Study the drawing (mm; zero at the part's minimum x, y, z) and answer. Coordinates: 2 decimals unless noted, no trailing zeros. Loops run counter-clockwise (first coordinate to the right, second up) from the corner with the lowest first, then second, coordinate; pieces in that order, holes last. Notation, with made-up numbers: (24, -31) -> (28, -31) arc R8 ccw to (28, -19) -> close; hole circle Ø2 at (3, 10.25). An arc over 180 degrees is marked (long way). Answer in a Markdown table with one row per item.
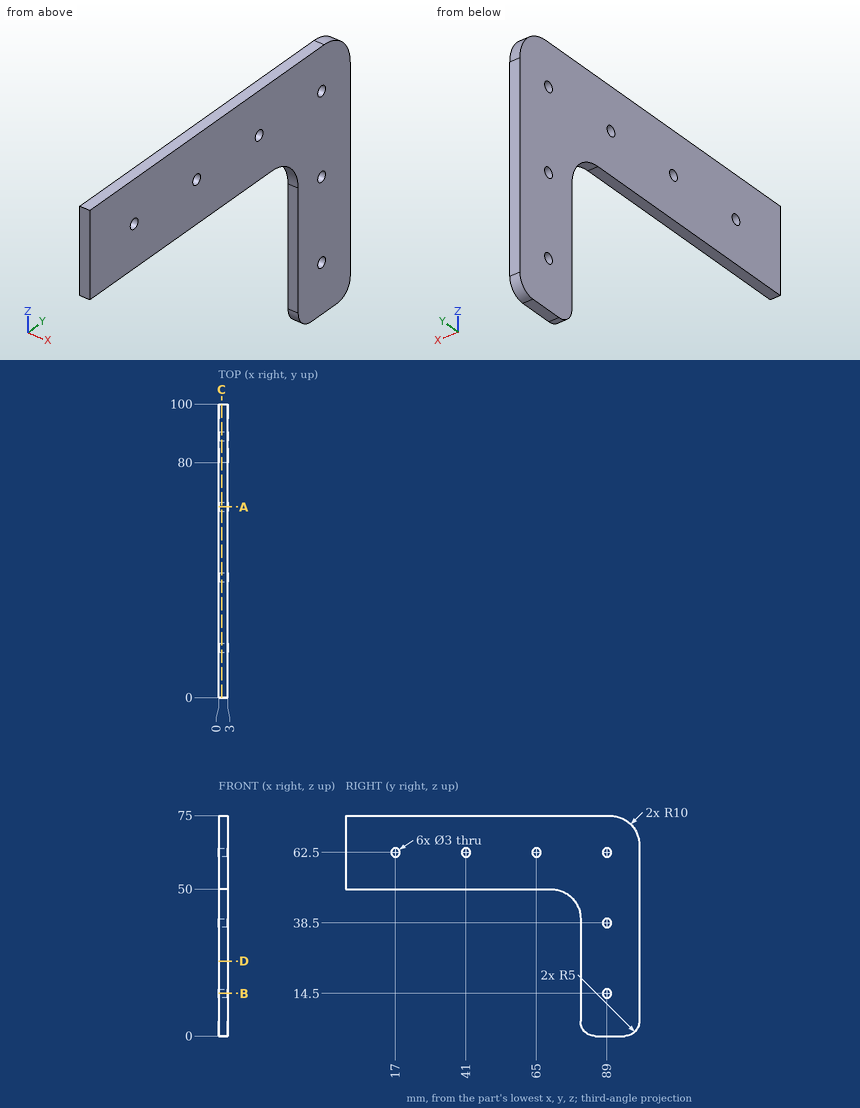
1. A cutting plane is placed at A-A on y = 65. Give the vertices of the cut face in (x, z), and give its area (3 significant figures).
A:
| item | result |
|---|---|
| outline | (0, 50) -> (3, 50) -> (3, 61) -> (0, 61) -> close; (0, 64) -> (3, 64) -> (3, 75) -> (0, 75) -> close |
| area | 66.0 mm2 |
2. Given pin 1 Ø1.8 at (y, z) = (89, 38.5) entering from -X; pin 2 Ø1 at (x, z) = (1.5, 29.5) entering from -Y, each flat-ended and moving along its own axis, determine where each tip first touches the part or whether it passes through.
A:
| item | result |
|---|---|
| pin 1 | passes through |
| pin 2 | stops at y = 80 |
3. A cutting plane is placed at D-D on z = 25.5. Give the vertices of the cut face in (x, y).
A:
| item | result |
|---|---|
| outline | (0, 80) -> (3, 80) -> (3, 100) -> (0, 100) -> close |
4. A cutting plane is placed at B-B on z = 14.5. Give the vertices of the cut face in (x, y).
A:
| item | result |
|---|---|
| outline | (0, 80) -> (3, 80) -> (3, 87.5) -> (0, 87.5) -> close; (0, 90.5) -> (3, 90.5) -> (3, 100) -> (0, 100) -> close |
5. Find the intervals of material crossed by probe 1 along Y at (x, z) = (0.9, 62.5); probe 2 along Z at (x, y) = (1.3, 89); probe 3 along Z at (x, y) = (1.45, 41), in increasing order.
A:
| item | result |
|---|---|
| probe 1 | y = 0 to 15.5, 18.5 to 39.5, 42.5 to 63.5, 66.5 to 87.5, 90.5 to 100 |
| probe 2 | z = 0 to 13, 16 to 37, 40 to 61, 64 to 75 |
| probe 3 | z = 50 to 61, 64 to 75 |
6. A cutting plane is placed at C-C on x = 1. Give the vertices of the cut face in (y, z).
A:
| item | result |
|---|---|
| outline | (0, 50) -> (70, 50) arc R10 cw to (80, 40) -> (80, 5) arc R5 ccw to (85, 0) -> (95, 0) arc R5 ccw to (100, 5) -> (100, 65) arc R10 ccw to (90, 75) -> (0, 75) -> close; hole circle Ø3 at (17, 62.5); hole circle Ø3 at (41, 62.5); hole circle Ø3 at (65, 62.5); hole circle Ø3 at (89, 14.5); hole circle Ø3 at (89, 38.5); hole circle Ø3 at (89, 62.5) |
